Read the model definition and answer for the solid it produces. Units are mm, in the model's axes. Face numbers are marked on the shaded views. Coordinates: 2 decimals unless noted, no trailing zeros. Order: outer loops, then holes, each group sorted by start corner. A loop starts at its lowest first (then second) coordinate and runs counter-clockwise, first axis right, second up. Notation, with made-up numbers: M -38.5,-1 L 1.5,-1 A22 ccw 1.5,22 Z; hole C 59.25,71 d5. An arc over 180 degrees is marked long. Use a Markdown table: item, result. Add a question column.
1) Find section D-D on y = 1.5. Write down the section's boundary in (x, z).
2) Find the intervals of material crossed by probe 1 along Z at (x, y) = (-15, 15); probe 2 along X at (y, z) = (8.75, -10); probe 3 along X at (y, z) = (8.5, -8), in increasing order. Write a range as [from, to].
3) Find section B-B on y = 14.5. Write down the section's boundary in (x, z), plus the area to 3 significant figures.
4) The mould has two halves that part along X. Classify the marked faces 1, 2, 3 and 4: released by +X, released by -X, zero draft, split by the parting line, or undercut.
5) Find section C-C on x = -15. Write down the section's boundary in (y, z).
6) Find section A-A on z = -10. Write down the section's boundary in (x, y).
7) Each of these flat-tipped pins is pushed along its axis until it touches: pin 1 Ø3 at (x, z) = (-15, -40) entering from +Y; pin 2 Ø2 at (x, z) = (-18.5, -7.5) entering from -Y. Where does it stop, or does it pass through?
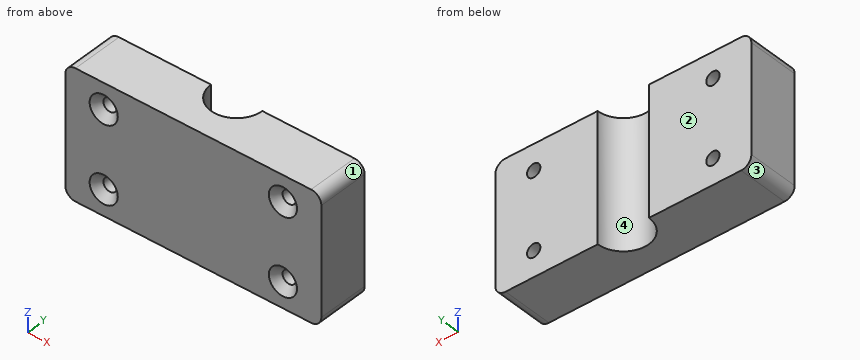
Autodesk Inventor part; units mm, degrees
ref_plane "YZ Plane" through (0, 0, 0) normal (1, 0, 0) x (0, 1, 0)
ref_plane "XZ Plane" through (0, 0, 0) normal (0, 1, 0) x (-1, 0, 0)
ref_plane "XY Plane" through (0, 0, 0) normal (0, 0, 1) x (1, 0, 0)
sketch "Skizze1" plane through (0, 0, 0) normal (0, 1, 0) x (-1, 0, 0)
  line L0 (0, 0) -> (0, -50)
  line L1 (0, -50) -> (100, -50)
  line L2 (100, -50) -> (100, 0)
  line L3 (100, 0) -> (0, 0)
  dimension "d0" = 50
  dimension "d1" = 100
extrude "Extrusion1" add sketch "Skizze1" along normal blind 20
fillet "Rundung1" radius 4 4 edges at (0, 10, 0) (0, 10, -50) (-100, 10, -50) (-100, 10, 0)
sketch "Skizze2" plane through (-96, 0, 0) normal (0, 0, 1) x (1, 0, 0)
  line L0 (0, 20) -> (0, 0)
  line L1 (0, 0) -> (46, 0)
  line L2 (0, 0) -> (92, 0)
  line L3 (46, 0) -> (46, 20)
  circle A0 centre (46, 20) radius 10
  point P0 (96, 0)
  dimension "d5" = 46
  dimension "d6" = 20
  dimension "d7" = 20
extrude "Extrusion2" cut sketch "Skizze2" against normal through all
sketch "Skizze3" plane through (0, 0, 0) normal (0, -1, 0) x (1, 0, 0)
  line L0 (0, 0) -> (0, -10)
  line L1 (0, -4) -> (0, -46)
  line L2 (0, -10) -> (-15, -10)
  line L3 (-15, -10) -> (-85, -10)
  line L4 (-85, -10) -> (-85, -40)
  line L5 (-85, -40) -> (-15, -40)
  dimension "d10" = 10
  dimension "d11" = 15
  dimension "d12" = 70
  dimension "d13" = 30
hole "Bohrung1" at (-85, 0, -40) at (-85, 0, -10) at (-15, 0, -40) at (-15, 0, -10) direction (0, 1, 0) diameter 5.2 end through all countersink diameter 11 countersink angle 90
equation "\"d0\" = breite"
equation "\"d1\" = länge"
equation "\"d4\" = radius"
equation "\"d7\" = durchmesser"
properties part number "TrittOT" material "PVC, hart"
Check result:
| question | item | result |
|---|---|---|
| 1 | outline | M -100,-46 A4 ccw -96,-50 L -4,-50 A4 ccw 0,-46 L 0,-4 A4 ccw -4,0 L -96,0 A4 ccw -100,-4 Z; hole C -85,-40 d8; hole C -85,-10 d8; hole C -15,-40 d8; hole C -15,-10 d8 |
| 2 | probe 1 | z = [-50, -42.6], [-37.4, -12.6], [-7.4, 0] |
| 2 | probe 2 | x = [-100, -87.6], [-82.4, -17.6], [-12.4, 0] |
| 2 | probe 3 | x = [-100, -86.66], [-83.34, -16.66], [-13.34, 0] |
| 3 | outline | M -100,-46 A4 ccw -96,-50 L -58.35,-50 L -58.35,0 L -96,0 A4 ccw -100,-4 Z; M -41.65,-50 L -4,-50 A4 ccw 0,-46 L 0,-4 A4 ccw -4,0 L -41.65,0 Z; hole C -85,-40 d5.2; hole C -85,-10 d5.2; hole C -15,-40 d5.2; hole C -15,-10 d5.2 |
| 3 | area | 4,070 mm2 |
| 4 | face 1 | released by +X |
| 4 | face 2 | zero draft |
| 4 | face 3 | released by -X |
| 4 | face 4 | undercut |
| 5 | outline | M 0,-50 L 20,-50 L 20,-42.6 L 2.9,-42.6 L 0,-45.5 Z; M 0,-34.5 L 2.9,-37.4 L 20,-37.4 L 20,-12.6 L 2.9,-12.6 L 0,-15.5 Z; M 0,-4.5 L 2.9,-7.4 L 20,-7.4 L 20,0 L 0,0 Z |
| 6 | outline | M -100,0 L -90.5,0 L -87.6,2.9 L -87.6,20 L -100,20 Z; M -82.4,2.9 L -79.5,0 L -20.5,0 L -17.6,2.9 L -17.6,20 L -40,20 A10 cw -60,20 L -82.4,20 Z; M -12.4,2.9 L -9.5,0 L 0,0 L 0,20 L -12.4,20 Z |
| 7 | pin 1 | passes through |
| 7 | pin 2 | stops at y = 0.2 |
